from build123d import *

# Parameters (mm, degrees)
F0_W     = 190
F0_H     = 106
F1_DEPTH = 0.8
F2_R     = 12.5
F3_DEPTH = 0.8


# Not quite as in the source:
# - a feature names something its author has since deleted; it is built from what else it names


with BuildPart() as f1:
    # F0 (on Top) → F1 (new body)
    with BuildSketch(Plane.XY):
        with Locations((-95, 53)):
            Rectangle(F0_W, F0_H)
    extrude(amount=F1_DEPTH)

    # F2 (on face) → F3 (join)
    with BuildSketch(Plane(origin=(0, 0, 0), x_dir=(1, 0, 0), z_dir=(0, 0, -1))):
        Circle(F2_R)
        with Locations((-190, 0)):
            Circle(F2_R)
        with Locations((-190, -106)):
            Circle(F2_R)
        with Locations((0, -106)):
            Circle(F2_R)
    extrude(amount=-F3_DEPTH)


solid = f1.part
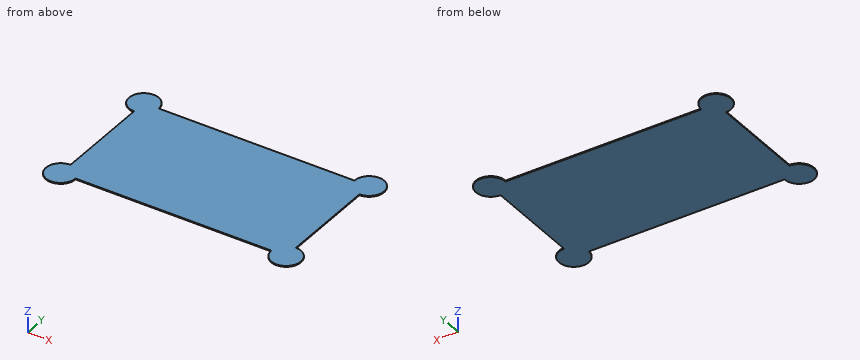
Source: CAD feature listing. Evaluate the final solid. Frame: model axes, mm. Round coordinates to 2 decimals unless told otherwise and drop trailing zeros. Loops run counter-clockwise (first coordinate to the right, second up) from the corner with the lowest first, then second, coordinate; pieces in that order, holes last. Notation, with made-up numbers: M 40.5,64.5 L 47.5,64.5 A21 ccw 47.5,90.5 Z; hole C -1,-13 d6. An arc over 180 degrees is marked long. Answer as CSV lines item,"result".
Q1. Cut plane C-C (x = -160.5). Return the cut outline in (y, z), plus the area to 3 significant figures.
Verdict:
outline,"M 0,0 L 106,0 L 106,0.8 L 0,0.8 Z"
area,"84.8 mm^2"
Q2. Cut plane A-A (z = 0.15). Return the cut outline in (x, y).
Verdict:
outline,"M -190,12.5 A12.5 ccw long -177.5,0 L -12.5,0 A12.5 ccw long 0,12.5 L 0,93.5 A12.5 ccw long -12.5,106 L -177.5,106 A12.5 ccw long -190,93.5 Z"
Q3. Cut plane B-B (y = 54.5). Return the cut outline in (x, z).
Verdict:
outline,"M -190,0 L 0,0 L 0,0.8 L -190,0.8 Z"
Q4. Line query: line 1 along Y through (x, z) = (-82, 0.1); line 2 along X through (y, z) = (29, 0.5); line 3 along Y through (x, z) = (3, 0.7). Output: solid intervals per line, ascending.
Verdict:
line 1,"y = 0 to 106"
line 2,"x = -190 to 0"
line 3,"y = -12.13 to 12.13, 93.87 to 118.13"
